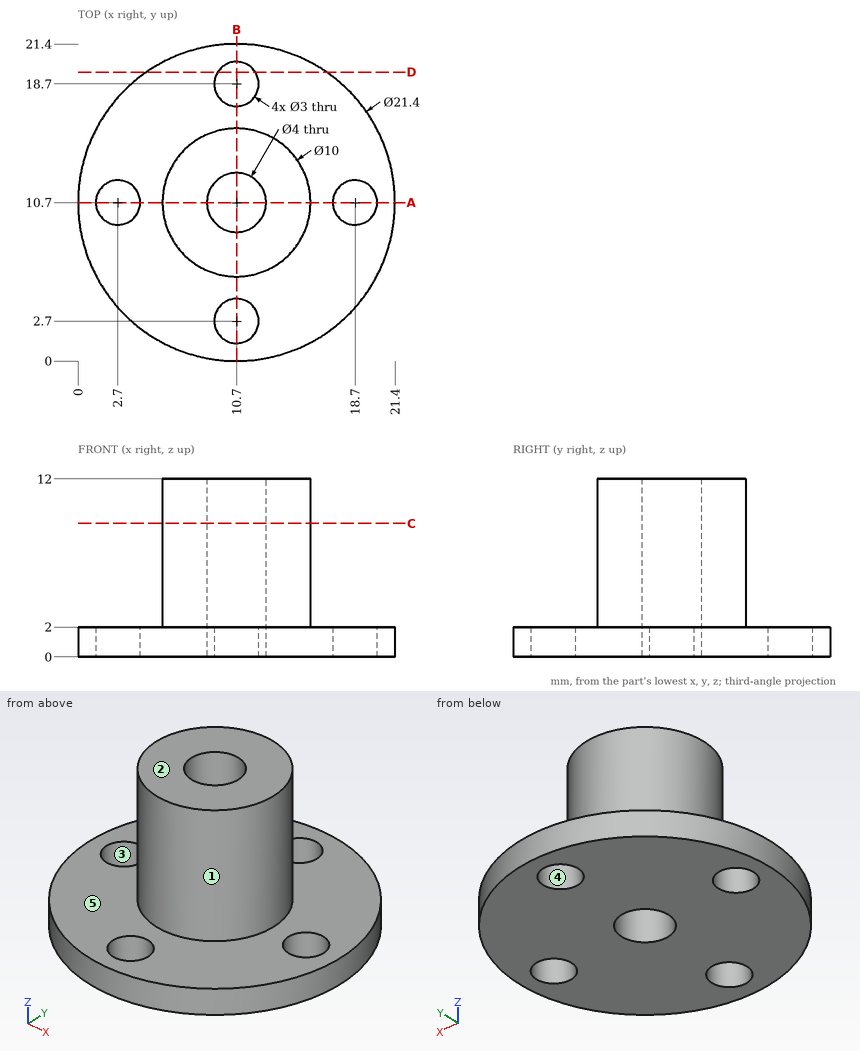
Input: dimensioned drawing with shaded views. Units: mm. Origin: part minimum x, y, z. A direction names the side the tool comes from. Coordinates: 2 decimals unless noted, no trailing zeros. Order: outer loops, then holes, each group sorted by start corner. A loop starts at its lowest first (then second) coordinate and runs counter-clockwise, first axis right, second up. Notation, with made-up numbers: (64, 26.5) - (109, 26.5) arc R18 ccw to (109, 43.5) - close; hole circle Ø9 at (86.25, 42.25). An arc over 180 degrees is marked (long way). Return JSON: item names as keys, results as strings. Group by question number.
1. Pin query (flat end, axial travel): pin 1 (5 mm diameter, centred on x = 18.7, y = 10.7, fed in from +Z); pin 2 (1.5 mm diameter, centred on x = 9.5, z = 3.5, fed in from -Y); pin 3 (5 mm diameter, centred on x = 2.5, z = 7, fed in from +Y); pin 4 (2 mm diameter, centred on x = 13, z = 7.5, fed in from +Y). Return the tip coordinate at first contact, or that it passes through.
2. Cut plane A-A (y = 10.7). Output: boundary loops of the cut face in (x, z).
3. Pull-direction query (X, two-part tool) for the marked faces 1, 2 and 3; classes: pulls with the +X half, pulls with the -X half, needs draft (parallel to the pull), parting line crosses it, or undercut.
4. Cut plane C-C (z = 9). Output: boundary loops of the cut face in (x, y), plus the area to 3 significant figures.
5. Material intervals for line 1 along Y through (x, z) = (10.7, 3); line 2 along Z through (x, y) = (13.75, 19); line 3 along Y through (x, z) = (18.5, 1), sorted ascending. Write a range as [from, to].
6. Cut plane D-D (y = 19.5). Output: boundary loops of the cut face in (x, z).
7. Set-up query: the marked faces 4 and 5. Return all of +Z, -Z, +X, -X, +Y, -Y with unobstructed straight access to the full face (end or side cutting, diameter ignored); none if empty.
Resolved:
{
 "1": {"pin 1": "stops at z = 2", "pin 2": "stops at y = 5.72", "pin 3": "passes through", "pin 4": "stops at y = 15.53"},
 "2": {"outline": "(0, 0) - (1.2, 0) - (1.2, 2) - (0, 2) - close; (4.2, 0) - (8.7, 0) - (8.7, 12) - (5.7, 12) - (5.7, 2) - (4.2, 2) - close; (12.7, 0) - (17.2, 0) - (17.2, 2) - (15.7, 2) - (15.7, 12) - (12.7, 12) - close; (20.2, 0) - (21.4, 0) - (21.4, 2) - (20.2, 2) - close"},
 "3": {"face 1": "parting line crosses it", "face 2": "needs draft", "face 3": "undercut"},
 "4": {"outline": "circle Ø10 at (10.7, 10.7); hole circle Ø4 at (10.7, 10.7)", "area": "66.0 mm²"},
 "5": {"line 1": "y = [5.7, 8.7], [12.7, 15.7]", "line 2": "z = [0, 2]", "line 3": "y = [3.38, 9.21], [12.19, 18.02]"},
 "6": {"outline": "(4.61, 0) - (9.43, 0) - (9.43, 2) - (4.61, 2) - close; (11.97, 0) - (16.79, 0) - (16.79, 2) - (11.97, 2) - close"},
 "7": {"face 4": "+Z, -Z", "face 5": "+Z"}
}
